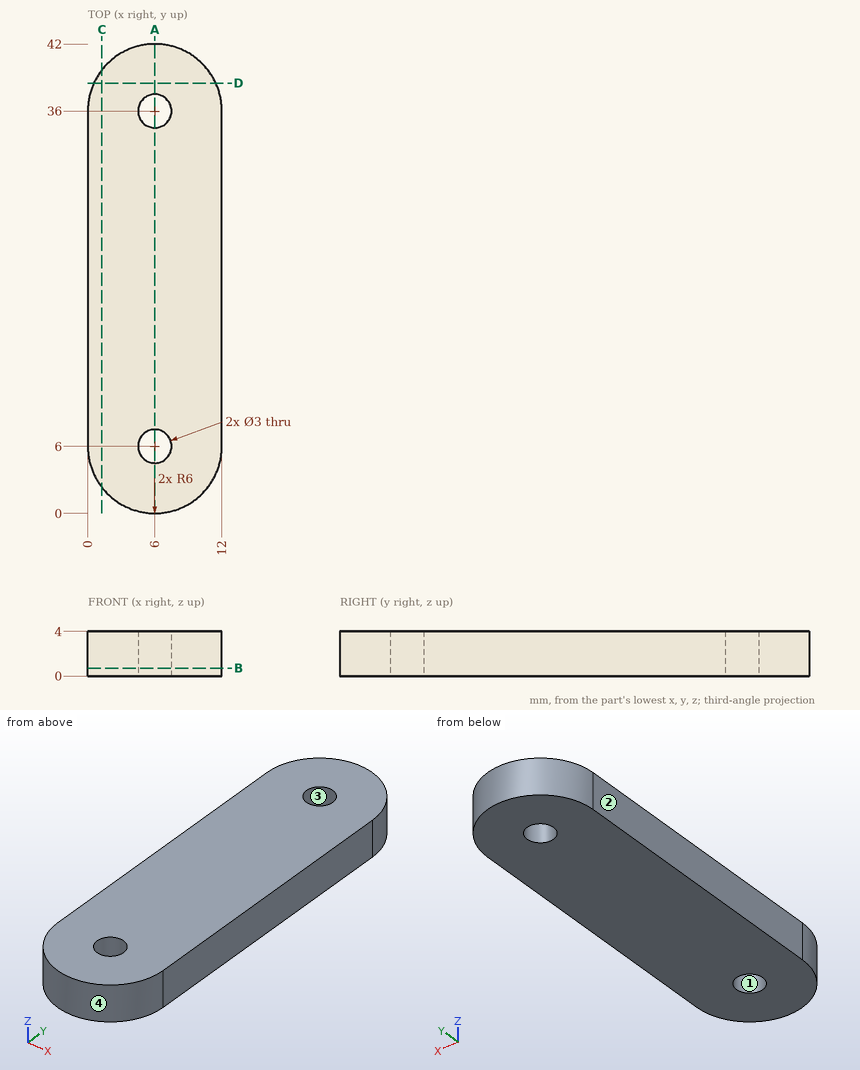
Answer from the drawing. Dimensions are ordinates in mm from the lowest x, y and z of the part. Round coordinates to 2 decimals unless told otherwise and drop trailing zeros. Write each loop counter-clockwise with the first axis right and the second up, starting at its lowest first coordinate (ties: lowest second). Pieces come first, ordered by that corner, then holes. Notation, with made-up numbers: M 50.25,16.25 L 86.25,16.25 A17 ccw 86.25,47.25 Z; hole C -29.75,40 d9. An arc over 180 degrees is marked long. Write each question's results on one line, items separated by ' | '. Start each with the question number.
Item 1: Flat-ended cylindrical pins translate along their axes: pin 1 Ø1 at (x, y) = (3.5, 8) entering from -Z; pin 2 Ø1.5 at (x, z) = (1.5, 2.5) entering from -Y. Find the tip coordinate at first contact, or state that the pin passes through.
Item 2: A cutting plane is placed at D-D on y = 38.5. Write down the section's boundary in (x, z).
Item 3: A cutting plane is placed at A-A on x = 6. Write down the section's boundary in (y, z), and give its area (3 significant figures).
Item 4: Straight lines are drawn through the part: L1, parallel to Y at x = 6, z = 1.8; L2, parallel to Y at x = 5.5, z = 1.2; L3, parallel to Y at x = 8.5, z = 1.8. For each, find the intervals that lie inside material, in ascending order. Write a range as [from, to].
Item 5: For a pull along X with two mould halves and no side action, classify the marked faces 1, 2, 3 and 4 as pulls with the +X half, pulls with the -X half, needs draft (parallel to the pull), parting line crosses it, or undercut.
Item 6: A cutting plane is placed at C-C on x = 1.25. Write down the section's boundary in (y, z).
Item 7: A cutting plane is placed at B-B on z = 0.7. Write down the section's boundary in (x, y).
Check sheet entries:
1) pin 1: z = 0 | pin 2: y = 1.32
2) outline: M 0.55,0 L 11.45,0 L 11.45,4 L 0.55,4 Z
3) outline: M 0,0 L 4.5,0 L 4.5,4 L 0,4 Z; M 7.5,0 L 34.5,0 L 34.5,4 L 7.5,4 Z; M 37.5,0 L 42,0 L 42,4 L 37.5,4 Z | area: 144 mm²
4) L1: [0, 4.5], [7.5, 34.5], [37.5, 42] | L2: [0.02, 4.59], [7.41, 34.59], [37.41, 41.98] | L3: [0.55, 41.45]
5) face 1: undercut | face 2: pulls with the -X half | face 3: undercut | face 4: parting line crosses it
6) outline: M 2.33,0 L 39.67,0 L 39.67,4 L 2.33,4 Z
7) outline: M 0,6 A6 ccw 12,6 L 12,36 A6 ccw 0,36 Z; hole C 6,6 d3; hole C 6,36 d3
